The listing builds one solid part. Answer for the finished solid, in the listing's coordinates (mm). A direction names the side the tool comes from. Round coordinates to 2 decimals unless told otherwise and drop trailing zeros. Write each loop counter-clockwise with the first axis right and the second up, starting at its lowest first coordinate (ties: lowest second). Pieces come first, ordered by that corner, then holes.
(1) A cutting plane is placed at A-A, the plane x = -5. Give the vertices of the cut face in (y, z), and give its area (3 significant figures).
(2) For faces 1 (the face through (10, 10, 1)), 2 (the face through (-6.1, 0, 2)), 3 (the face through (-7, 0, 0)), determine the directions among +Z, -Z, +X, -X, +Y, -Y from which every point of the face is accessible in a straight line to the end or side of a thin tool.
(3) Each of these flat-tipped pins is pushed along its axis until it touches: pin 1 Ø4 at (x, y) = (7.5, -4) entering from -Z; pin 2 Ø3 at (x, z) = (5, -6) entering from +Y; pin 3 Ø10 at (x, z) = (3.5, -16) entering from -Y. Where does it stop, or does it pass through?
(4) A cutting plane is placed at B-B, the plane z = -6. Give the vertices of the cut face in (x, y).
(5) Find the intervals of material crossed by probe 1 along X at (y, z) = (20.2, -6); probe 2 along Y at (x, z) = (0, 3.2); probe 3 along Z at (x, y) = (5, 20), in increasing order.
(6) The mould has two halves that part along Z. Classify faces 4 (the face through (0, 20, -26)), 5 (the face through (0, 11.35, 2)), 6 (the face through (-5.228, 20.035, -21.735)): +Z half, -Z half, draft (parallel to the pull), parting line (faces both ways), or undercut.
(7) A cutting plane is placed at C-C, the plane y = 18. Give the vertices of the cut face in (x, z), and give its area (3 significant figures).
(8) A cutting plane is placed at D-D, the plane y = 9.5. Give the vertices of the cut face in (x, z), and give its area (3 significant figures).
from build123d import *

# Parameters (mm, degrees)
SKETCH1_W           = 20
SKETCH1_H           = 45
BOSS_EXTRUDE1_DEPTH = 4.2
SKETCH2_W           = 12.2
SKETCH2_H           = 22.7
CUT_EXTRUDE1_DEPTH  = 5
SKETCH3_R           = 1
SKETCH3_R_2         = 1.001337469
CUT_EXTRUDE2_DEPTH  = 5
SKETCH4_W           = 20
SKETCH4_H           = 5
BOSS_EXTRUDE2_DEPTH = 26
SKETCH5_R           = 1.75
CUT_EXTRUDE3_DEPTH  = 15
SKETCH6_W           = 20
SKETCH6_H           = 5
CUT_EXTRUDE4_DEPTH  = 15


with BuildPart() as part:
    # Sketch1 → Boss-Extrude1 (new body)
    with BuildSketch(Plane.XY):
        Rectangle(SKETCH1_W, SKETCH1_H)
    extrude(amount=BOSS_EXTRUDE1_DEPTH)

    # Sketch2 → Cut-Extrude1 (cut)
    with BuildSketch(Plane(origin=(0, 0, 0), x_dir=(-1, 0, 0), z_dir=(0, 0, -1))):
        Rectangle(SKETCH2_W, SKETCH2_H)
    extrude(amount=-CUT_EXTRUDE1_DEPTH, mode=Mode.SUBTRACT)

    # Sketch3 → Cut-Extrude2 (cut)
    with BuildSketch(Plane.XY.offset(4.2)):
        with Locations((0, 14.4)):
            Circle(SKETCH3_R)
        with Locations((0, -14.396360879)):
            Circle(SKETCH3_R_2)
    extrude(amount=-CUT_EXTRUDE2_DEPTH, mode=Mode.SUBTRACT)

    # Sketch4 → Boss-Extrude2 (add)
    with BuildSketch(Plane(origin=(0, 0, 0), x_dir=(-1, 0, 0), z_dir=(0, 0, -1))):
        with Locations((0, 20)):
            Rectangle(SKETCH4_W, SKETCH4_H)
    extrude(amount=BOSS_EXTRUDE2_DEPTH)

    # Sketch5 → Cut-Extrude3 (cut)
    with BuildSketch(Plane(origin=(0, 22.5, 0), x_dir=(1, 0, 0), z_dir=(0, 1, 0))):
        with Locations((-5, 6)):
            Circle(SKETCH5_R)
        with Locations((5, 6)):
            Circle(SKETCH5_R)
        with Locations((5, 20)):
            Circle(SKETCH5_R)
        with Locations((-5, 20)):
            Circle(SKETCH5_R)
    extrude(amount=-CUT_EXTRUDE3_DEPTH, mode=Mode.SUBTRACT)

    # Sketch6 → Cut-Extrude4 (cut)
    with BuildSketch(Plane.XY.offset(4.2)):
        with Locations((0, -20)):
            Rectangle(SKETCH6_W, SKETCH6_H)
    extrude(amount=-CUT_EXTRUDE4_DEPTH, mode=Mode.SUBTRACT)


solid = part.part
Solutions:
1. outline: (-17.5, 0) - (-11.35, 0) - (-11.35, 4.2) - (-17.5, 4.2) - close; (11.35, 0) - (17.5, 0) - (17.5, -4.25) - (22.5, -4.25) - (22.5, 4.2) - (11.35, 4.2) - close; (17.5, -26) - (22.5, -26) - (22.5, -21.75) - (17.5, -21.75) - close; (17.5, -18.25) - (22.5, -18.25) - (22.5, -7.75) - (17.5, -7.75) - close
1. area: 168 mm2
2. face 1: +Z, -Z, +X, +Y, -Y
2. face 2: +Z, -Z
2. face 3: -Z, +X, -X, -Y
3. pin 1: stops at z = 0
3. pin 2: passes through
3. pin 3: stops at y = 17.5
4. outline: (-10, 17.5) - (-6.75, 17.5) - (-6.75, 22.5) - (-10, 22.5) - close; (-3.25, 17.5) - (3.25, 17.5) - (3.25, 22.5) - (-3.25, 22.5) - close; (6.75, 17.5) - (10, 17.5) - (10, 22.5) - (6.75, 22.5) - close
5. probe 1: x = -10 to -6.75, -3.25 to 3.25, 6.75 to 10
5. probe 2: y = -17.5 to -15.4, -13.4 to -11.35, 11.35 to 13.4, 15.4 to 22.5
5. probe 3: z = -26 to -21.75, -18.25 to -7.75, -4.25 to 4.2
6. face 4: -Z half
6. face 5: draft
6. face 6: undercut
7. outline: (-10, -26) - (10, -26) - (10, 4.2) - (-10, 4.2) - close; hole circle Ø3.5 at (-5, -20); hole circle Ø3.5 at (-5, -6); hole circle Ø3.5 at (5, -20); hole circle Ø3.5 at (5, -6)
7. area: 566 mm2
8. outline: (-10, 0) - (-6.1, 0) - (-6.1, 4.2) - (-10, 4.2) - close; (6.1, 0) - (10, 0) - (10, 4.2) - (6.1, 4.2) - close
8. area: 32.8 mm2
